```python
from build123d import *

# Parameters (mm, degrees)
SKETCH1_W                                     = 15
SKETCH1_H                                     = 8
CBORE_FOR_M3_HEX_HEAD_MACHINE_SCREW1_AT_COUNT = 2
CBORE_FOR_M3_HEX_HEAD_MACHINE_SCREW1_AT_PITCH = 81.99963788
CBORE_FOR_M3_HEX_HEAD_MACHINE_SCREW1_2_COUNT  = 2
CBORE_FOR_M3_HEX_HEAD_MACHINE_SCREW1_2_PITCH  = 81.99963788
CBORE_FOR_M3_HEX_HEAD_MACHINE_SCREW1_3_COUNT  = 2
CBORE_FOR_M3_HEX_HEAD_MACHINE_SCREW1_3_PITCH  = 115.965


with BuildPart() as part:
    # Sketch1 → Revolve1 (revolve)
    with BuildSketch(Plane.XY, mode=Mode.PRIVATE) as revolve1_sk:
        with Locations((55.1885, 4)):
            Rectangle(SKETCH1_W, SKETCH1_H)
    revolve(revolve1_sk.sketch.rotate(Axis((0, 0, 0), (0, 1, 0)), 90), axis=Axis((0, 0, 0), (0, 1, 0)))

    # Sketch3 → CBORE for M3 Hex Head Machine Screw1 (revolve, cut)
    with BuildSketch(Plane(origin=(0, 0, -57.9825), x_dir=(0, 0, -1), z_dir=(1, 0, 0))):
        Polygon((0, 0), (0, 8), (1.7, 8), (1.7, 2.3), (4.2, 2.3), (4.2, 0.025), (4.225, 0), align=None)
    cbore_for_m3_hex_head_machine_screw1 = revolve(axis=Axis((0, -6.35, -57.9825), (0, 1, 0)), mode=Mode.SUBTRACT)

    # CBORE for M3 Hex Head Machine Screw1 at: CBORE for M3 Hex Head Machine Screw1 ×2
    with Locations(*[Vector(0.7071067811865476, 0, 0.7071067811865476) * (i * CBORE_FOR_M3_HEX_HEAD_MACHINE_SCREW1_AT_PITCH) for i in range(1, CBORE_FOR_M3_HEX_HEAD_MACHINE_SCREW1_AT_COUNT)]):
        add(cbore_for_m3_hex_head_machine_screw1, mode=Mode.SUBTRACT)

    # CBORE for M3 Hex Head Machine Screw1 2: CBORE for M3 Hex Head Machine Screw1 ×2
    with Locations(*[Vector(-0.7071067811865476, 0, 0.7071067811865476) * (i * CBORE_FOR_M3_HEX_HEAD_MACHINE_SCREW1_2_PITCH) for i in range(1, CBORE_FOR_M3_HEX_HEAD_MACHINE_SCREW1_2_COUNT)]):
        add(cbore_for_m3_hex_head_machine_screw1, mode=Mode.SUBTRACT)

    # CBORE for M3 Hex Head Machine Screw1 3: CBORE for M3 Hex Head Machine Screw1 ×2
    with Locations(*[(0, 0, i * CBORE_FOR_M3_HEX_HEAD_MACHINE_SCREW1_3_PITCH) for i in range(1, CBORE_FOR_M3_HEX_HEAD_MACHINE_SCREW1_3_COUNT)]):
        add(cbore_for_m3_hex_head_machine_screw1, mode=Mode.SUBTRACT)


solid = part.part
```
CAD build for the part. Positions are in the model's coordinates, mm. A direction names the side the tool comes from. Give positions to 0.01 mm unless a question says otherwise; leave off trailing zeros. Loops run counter-clockwise (first coordinate to the right, second up) from the corner with the lowest first, then second, coordinate; pieces in that order, holes last. Notation, with made-up numbers: (47.5, -28.5) - (69.5, -28.5) arc R37 cw to (69.5, 9.5) - close; hole circle Ø11 at (49, -21.75). An arc over 180 degrees is marked (long way). Put each result on its own line as item: value.
Q1. Flat gauge pins, fed straight in: pin 1 (3 mm diameter, centred on y = 3, z = 28, fed in from -X); pin 2 (1.5 mm diameter, centred on y = 2.5, z = -12, fed in from -X); pin 3 (7.5 mm diameter, centred on x = 0, z = -57.98, fed in from -Y). Where does each tip first touch, or does it go through?
Filled in:
pin 1: stops at x = -56.81
pin 2: stops at x = -61.67
pin 3: stops at y = 2.3
Q2. Slice it at C-C (z = -29.5). Give the cut face in (x, y), plus the area to 3 significant figures.
Filled in:
outline: (-55.31, 0) - (-37.47, 0) - (-37.47, 8) - (-55.31, 8) - close; (37.47, 0) - (55.31, 0) - (55.31, 8) - (37.47, 8) - close
area: 286 mm²
Q3. Slice it at A-A (z = 0). Give the number of separate pieces and of enclosed holes in the cut face, plus the area to 3 significant figures.
Filled in:
separate pieces: 4
enclosed holes: 0
area: 163 mm²
Q4. Mould opens along Z. For faces 3 (the face through (-56, 2.3, 0)), 4 (the face through (23, 0, -42)), 5 (the face through (61.198, 4.056, 13.59)) say: pulls with the +Z half, pulls with the -Z half, needs draft (parallel to the pull), parting line crosses it, or undercut.
Filled in:
face 3: undercut
face 4: needs draft
face 5: parting line crosses it
Q5. Slice it at D-D (x = 13). Give the cut face in (y, z).
Filled in:
outline: (0, -61.33) - (8, -61.33) - (8, -45.88) - (0, -45.88) - close; (0, 45.88) - (8, 45.88) - (8, 61.33) - (0, 61.33) - close
Q6. Probe line 1 along X through (y, z) = (4.75, 0); line 2 along X through (y, z) = (0.75, 0); line 3 along Z through (x, y) = (-0.5, 2.5). List the from-to ranges inside material, lowest first.
Filled in:
line 1: x = -62.69 to -59.68, -56.28 to -47.69, 47.69 to 56.28, 59.68 to 62.69
line 2: x = -62.69 to -62.18, -53.78 to -47.69, 47.69 to 53.78, 62.18 to 62.69
line 3: z = -62.69 to -59.61, -56.36 to -47.69, 47.69 to 56.36, 59.61 to 62.69
Q7. Tool access for faces 1 (the face through (59.64, 5.11, 0.37)), 2 (the face through (53.82, 1.15, 0.55)): list every direction of +Z, -Z, +X, -X, +Y, -Y with a clear straight run to the whole face (end or side of a thin tool).
Filled in:
face 1: +Y, -Y
face 2: -Y
